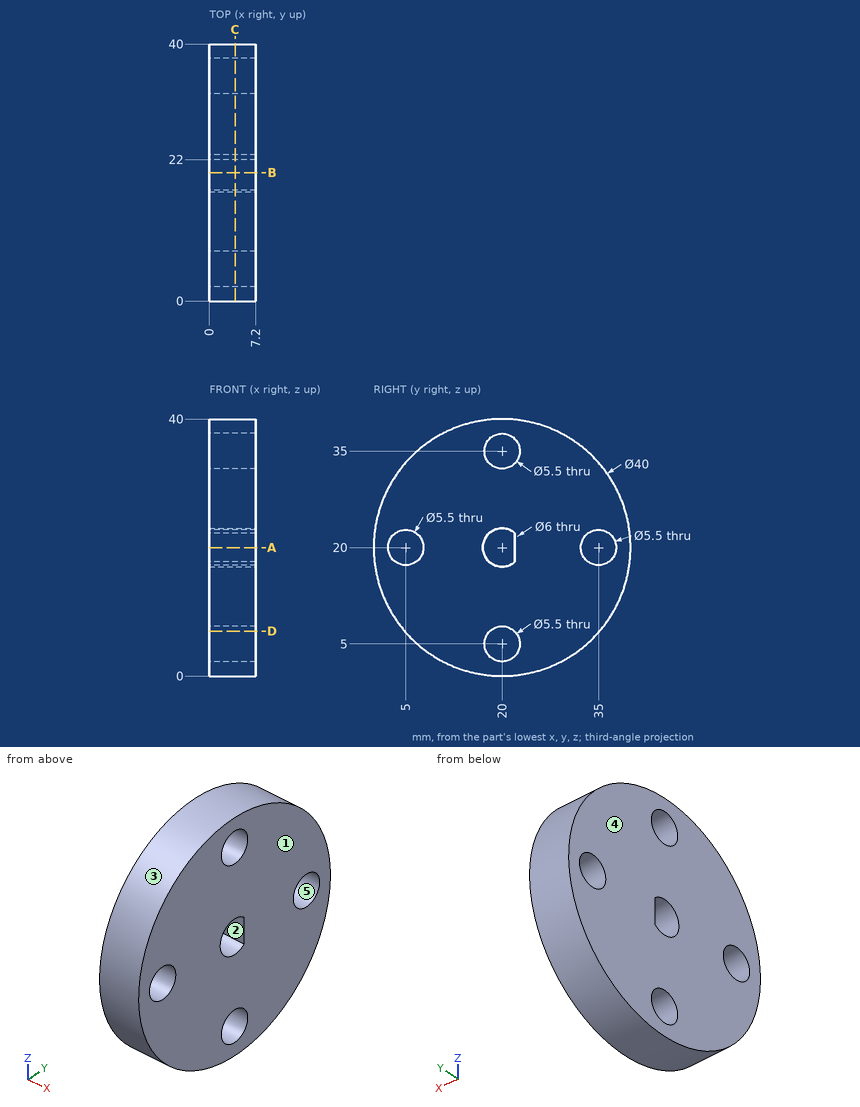
Check sheet for the drawn part. Datum: minimum x, y, z corner. Units: mm. A direction names the side the tool comes from. Round coordinates to 2 decimals unless told otherwise and drop trailing zeros. Order: outer loops, then holes, each group sorted by start corner. A loop starts at its lowest first (then second) coordinate and runs counter-clockwise, first axis right, second up.
(1) Scan lines: probe 1 along Y at (x, z) = (2.5, 20); probe 2 along Z at (x, y) = (4.75, 20.5); probe 3 along Z at (x, y) = (4.25, 18.5). Record each from-to range of solid material in increasing order.
(2) Access from +Z, -Z, +X, -X, +Y, -Y to the whole of each face (thin tool, end or side, straight path). Record for the marked faces 1 and 2.
(3) Cross-section at D-D, the plane z = 7. Enter the section's corners in (x, y), and give its area (3 significant figures).
(4) Draft check along Z on the marked faces 3, 4 and 5. Enter one of: pulls with the +Z half, pulls with the -Z half, needs draft (parallel to the pull), parting line crosses it, or undercut.
(5) Cross-section at A-A, the plane z = 20. Enter the section's corners in (x, y), and give its area (3 significant figures).
(6) Go/stop test with flat-tipped pins: P1, Ø1.3, axis at x = 5, z = 19, coming from the -Y side; P2, Ø4, axis at x = 3, z = 32.5, coming from the -Y side; P3, Ø2, axis at x = 4.5, z = 35.5, coming from the -Y side (3 decimals). Record where each tip stops, or that it passes through.
(7) Cross-section at B-B, the plane y = 20. Enter the section's corners in (x, z).
(8) Cross-section at C-C, the plane x = 4. Enter the section's corners in (y, z).
Check sheet entries:
1. probe 1: y = 0 to 2.25, 7.75 to 17, 22 to 32.25, 37.75 to 40
1. probe 2: z = 0.01 to 2.3, 7.7 to 17.04, 22.96 to 32.3, 37.7 to 39.99
1. probe 3: z = 0.06 to 2.7, 7.3 to 17.4, 22.6 to 32.7, 37.3 to 39.94
2. face 1: +Z, -Z, +X, +Y, -Y
2. face 2: +X, -X
3. outline: (0, 4.8) - (7.2, 4.8) - (7.2, 18.11) - (0, 18.11) - close; (0, 21.89) - (7.2, 21.89) - (7.2, 35.2) - (0, 35.2) - close
3. area: 192 mm2
4. face 3: parting line crosses it
4. face 4: needs draft
4. face 5: undercut
5. outline: (0, 0) - (7.2, 0) - (7.2, 2.25) - (0, 2.25) - close; (0, 7.75) - (7.2, 7.75) - (7.2, 17) - (0, 17) - close; (0, 22) - (7.2, 22) - (7.2, 32.25) - (0, 32.25) - close; (0, 37.75) - (7.2, 37.75) - (7.2, 40) - (0, 40) - close
5. area: 173 mm2
6. P1: stops at y = 0
6. P2: stops at y = 2.98
6. P3: stops at y = 6.225
7. outline: (0, 0) - (7.2, 0) - (7.2, 2.25) - (0, 2.25) - close; (0, 7.75) - (7.2, 7.75) - (7.2, 17) - (0, 17) - close; (0, 23) - (7.2, 23) - (7.2, 32.25) - (0, 32.25) - close; (0, 37.75) - (7.2, 37.75) - (7.2, 40) - (0, 40) - close
8. outline: circle Ø40 at (20, 20); hole circle Ø5.5 at (5, 20); hole circle Ø5.5 at (20, 5); hole circle Ø5.5 at (20, 35); hole (22, 17.76) - (22, 22.24) arc R3 ccw (long way) to start; hole circle Ø5.5 at (35, 20)
